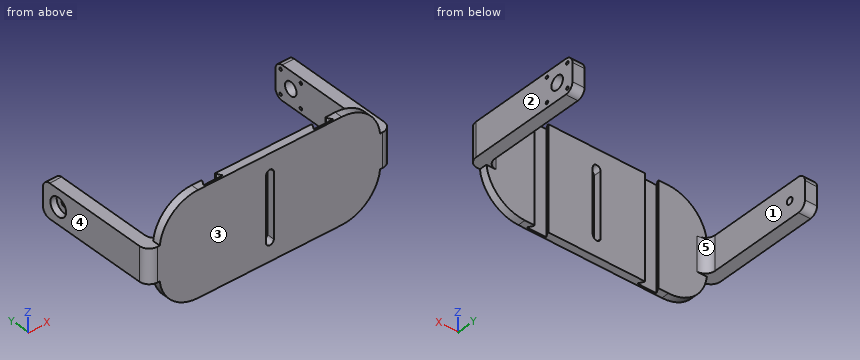
from build123d import *

# Parameters (mm, degrees)
SKETCH1_W           = 12.5
SKETCH1_H           = 127
BOSS_EXTRUDE1_DEPTH = 106
SKETCH2_W           = 12.5
SKETCH2_H           = 35.5
CUT_EXTRUDE1_DEPTH  = 200
SKETCH4_4_R         = 6
CUT_EXTRUDE3_DEPTH  = 37
SKETCH4_R           = 7
SKETCH4_R_2         = 1.55
CUT_EXTRUDE4_DEPTH  = 18.375
FILLET3_R           = 8
FILLET4_R           = 10
FILLET5_R           = 40
SKETCH5_R           = 3.5
CUT_EXTRUDE5_DEPTH  = 25
CUT_EXTRUDE6_START  = -6
SKETCH5_3_R         = 9.5
SKETCH5_3_R_2       = 3.5
CUT_EXTRUDE6_DEPTH  = 7


with BuildPart() as part:
    # Sketch1 → Boss-Extrude1 (new body)
    with BuildSketch(Plane.XY):
        Polygon((0, 8), (0, 0), (228, 0), (228, 8), (178.113248654, 8), (178.113248654, 7), (181, 2), (161, 2), (163.886751346, 7), (163.886751346, 8), (64.113248654, 8), (64.113248654, 7), (67, 2), (47, 2), (49.886751346, 7), (49.886751346, 8), align=None)
        with Locations((234.25, 63.5)):
            Rectangle(SKETCH1_W, SKETCH1_H)
        with Locations((-6.25, 63.5)):
            Rectangle(SKETCH1_W, SKETCH1_H)
    extrude(amount=-BOSS_EXTRUDE1_DEPTH)

    # Sketch2 → Cut-Extrude1 (cut)
    with BuildSketch(Plane(origin=(0, 127, 0), x_dir=(1, 0, 0), z_dir=(0, 1, 0))):
        with Locations((-6.25, 88.25)):
            Rectangle(SKETCH2_W, SKETCH2_H)
        with Locations((-6.25, 17.75)):
            Rectangle(SKETCH2_W, SKETCH2_H)
        with Locations((234.25, 88.25)):
            Rectangle(SKETCH2_W, SKETCH2_H)
        with Locations((234.25, 17.75)):
            Rectangle(SKETCH2_W, SKETCH2_H)
        with BuildLine():
            Line((109.95, 20), (109.95, 86))
            ThreePointArc((109.95, 86), (114, 90.05), (118.05, 86))
            Line((118.05, 86), (118.05, 20))
            ThreePointArc((118.05, 20), (114, 15.95), (109.95, 20))
        make_face()
    extrude(amount=-CUT_EXTRUDE1_DEPTH, mode=Mode.SUBTRACT)

    # Sketch4<4> → Cut-Extrude3 (cut)
    with BuildSketch(Plane(origin=(240.5, 0, 0), x_dir=(0, 0, -1), z_dir=(1, 0, 0))):
        with Locations((53, 108.5)):
            Circle(SKETCH4_4_R)
    extrude(amount=-CUT_EXTRUDE3_DEPTH, mode=Mode.SUBTRACT)

    # Sketch4 → Cut-Extrude4 (cut)
    with BuildSketch(Plane(origin=(240.5, 0, 0), x_dir=(0, 0, -1), z_dir=(1, 0, 0))):
        with Locations((53, 108.5)):
            Circle(SKETCH4_R)
        with Locations((40.625, 120.875)):
            Circle(SKETCH4_R_2)
        with Locations((40.625, 96.125)):
            Circle(SKETCH4_R_2)
        with Locations((65.375, 96.125)):
            Circle(SKETCH4_R_2)
        with Locations((65.375, 120.875)):
            Circle(SKETCH4_R_2)
    extrude(amount=-CUT_EXTRUDE4_DEPTH, mode=Mode.SUBTRACT)

    # Fillet3
    fillet3_edges = [part.edges().sort_by_distance(p)[0] for p in [
        (-6.25, 127, -35.5),
        (234.25, 127, -70.5),
        (234.25, 127, -35.5),
        (-6.25, 127, -70.5),
    ]]
    fillet(fillet3_edges, radius=FILLET3_R)

    # Fillet4
    fillet4_edges = [part.edges().sort_by_distance(p)[0] for p in [
        (228, 8, -53),
        (240.5, 0, -53),
        (0, 8, -53),
        (-12.5, 0, -53),
    ]]
    fillet(fillet4_edges, radius=FILLET4_R)

    # Fillet5
    # the kernel refuses this fillet: 40 mm, written as the material it takes off along each edge
    with BuildSketch(Plane(origin=(228, 107.36517247, -106), x_dir=(-1, 0, 0), z_dir=(0, -1, 0))) as fillet5_piece_1:
        with BuildLine():
            CenterArc((39.746068988, -40), FILLET5_R, 90, 83.540550223)
            Line((0, -35.5), (-0.79492138, -35.41))
            ThreePointArc((-0.79492138, -35.41), (-0.8, -17.75), (-0.8, 0))
            Line((-0.8, 0), (0, 0.8))
            Line((0, 0.8), (39.746068988, 0.8))
            Line((39.746068988, 0.8), (39.746068988, 0))
        make_face()
    extrude(amount=206.73034494, mode=Mode.SUBTRACT)
    with BuildSketch(Plane(origin=(0, 107.36517247, -106), x_dir=(0, 0, 1), z_dir=(0, -1, 0))) as fillet5_piece_2:
        with BuildLine():
            CenterArc((40, -39.746068988), FILLET5_R, 96.459449777, 83.540550223)
            Line((0, -39.746068988), (-0.8, -39.746068988))
            Line((-0.8, -39.746068988), (-0.8, 0))
            Line((-0.8, 0), (0, 0.8))
            ThreePointArc((0, 0.8), (17.75, 0.8), (35.41, 0.79492138))
            Line((35.41, 0.79492138), (35.5, 0))
        make_face()
    extrude(amount=206.73034494, mode=Mode.SUBTRACT)
    with BuildSketch(Plane(origin=(0, 107.36517247, 0), x_dir=(0, 0, -1), z_dir=(0, -1, 0))) as fillet5_piece_3:
        with BuildLine():
            CenterArc((40, 39.746068988), FILLET5_R, 180, 83.540550223)
            Line((0, 39.746068988), (-0.8, 39.746068988))
            Line((-0.8, 39.746068988), (-0.8, 0))
            Line((-0.8, 0), (0, -0.8))
            ThreePointArc((0, -0.8), (17.75, -0.8), (35.41, -0.79492138))
            Line((35.41, -0.79492138), (35.5, 0))
        make_face()
    extrude(amount=206.73034494, mode=Mode.SUBTRACT)
    with BuildSketch(Plane(origin=(228, 107.36517247, 0), x_dir=(-1, 0, 0), z_dir=(0, -1, 0))) as fillet5_piece_4:
        with BuildLine():
            CenterArc((39.746068988, 40), FILLET5_R, 186.459449777, 83.540550223)
            Line((0, 35.5), (-0.79492138, 35.41))
            ThreePointArc((-0.79492138, 35.41), (-0.8, 17.75), (-0.8, 0))
            Line((-0.8, 0), (0, -0.8))
            Line((0, -0.8), (39.746068988, -0.8))
            Line((39.746068988, -0.8), (39.746068988, 0))
        make_face()
    extrude(amount=206.73034494, mode=Mode.SUBTRACT)

    # Sketch5 → Cut-Extrude5 (cut)
    with BuildSketch(Plane(origin=(0, 0, 0), x_dir=(0, 0, -1), z_dir=(1, 0, 0))):
        with Locations((53, 108.5)):
            Circle(SKETCH5_R)
    extrude(amount=-CUT_EXTRUDE5_DEPTH, mode=Mode.SUBTRACT)

    # Sketch5<3> → Cut-Extrude6 (cut)
    with BuildSketch(Plane(origin=(0, 0, 0), x_dir=(0, 0, -1), z_dir=(1, 0, 0)).offset(CUT_EXTRUDE6_START)):
        with Locations((53, 108.5)):
            Circle(SKETCH5_3_R)
        with Locations((53, 108.5)):
            Circle(SKETCH5_3_R_2, mode=Mode.SUBTRACT)
    extrude(amount=-CUT_EXTRUDE6_DEPTH, mode=Mode.SUBTRACT)


solid = part.part
Geometry check sheet. Reference: the model listing, model coordinates, mm. Face numbers are marked on the shaded views. A direction names the side the tool comes from. Round coordinates to 2 decimals unless told otherwise and drop trailing zeros. Loops run counter-clockwise (first coordinate to the right, second up) from the corner with the lowest first, then second, coordinate; pieces in that order, holes last.
Item 1: Thickness scan on line 1 (Z direction, x = 233, y = 108); line 2 (X direction, y = 38, z = -65); line 3 (Y direction, x = 167, z = -45). Record the ranges inside material, lowest first.
Item 2: Cross-section at C-C on z = -74.5. Record the boundary of the cut face in (x, y), then the cut area to 3 significant figures.
Item 3: Access from +Z, -Z, +X, -X, +Y, -Y to the whole of each face (thin tool, end or side, straight path). Record for the marked faces 4 and 5.
Item 4: Cross-section at D-D on z = -53. Count the separate pieces of the cut face and the enclosed holes in it, then the cut area to 3 significant figures.
Item 5: Cross-section at A-A on y = 108.5. Record the boundary of the cut face in (x, z).
Item 6: Cross-section at B-B on x = 114. Record the boundary of the cut face in (y, z).
Item 7: Gauge pin test, flat ends, axial feed: pin 1 (15 mm diameter, centred on x = 207, z = -47, fed in from +Y); pin 2 (25 mm diameter, centred on x = 4, y = 75.5, fed in from -Z); pin 3 (6.5 mm diameter, centred on y = 108.5, z = -53, fed in from -X); pin 4 (18 mm diameter, centred on x = -1, y = 79, fed in from +Z). Record the tip position at first contact, or that the pin passes through.
Item 8: Mould release check, pull along X, two halves, no side actions. Record for the marked faces 1, 2 and 3: pulls with the +X half, pulls with the -X half, needs draft (parallel to the pull), parting line crosses it, or undercut.
Answer sheet:
1. line 1: z = -70.5 to -59.98, -46.02 to -35.5
1. line 2: x = -12.5 to 0, 228 to 240.5
1. line 3: y = 0 to 2
2. outline: (0.66, 0) - (109.95, 0) - (109.95, 8) - (64.11, 8) - (64.11, 7) - (67, 2) - (47, 2) - (49.89, 7) - (49.89, 8) - (0.66, 8) - close; (118.05, 0) - (227.34, 0) - (227.34, 8) - (178.11, 8) - (178.11, 7) - (181, 2) - (161, 2) - (163.89, 7) - (163.89, 8) - (118.05, 8) - close
2. area: 1,550 mm2
3. face 4: +Z, -Z, -X, +Y, -Y
3. face 5: +Z, -Z, +Y
4. separate pieces: 4
4. enclosed holes: 0
4. area: 4,390 mm2
5. outline: (-12.5, -70.5) - (0, -70.5) - (0, -56.5) - (-6, -56.5) - (-6, -62.5) - (-12.5, -62.5) - close; (-12.5, -43.5) - (-6, -43.5) - (-6, -49.5) - (0, -49.5) - (0, -35.5) - (-12.5, -35.5) - close; (228, -70.5) - (240.5, -70.5) - (240.5, -60) - (228, -60) - close; (228, -46) - (240.5, -46) - (240.5, -35.5) - (228, -35.5) - close
6. outline: (0, -106) - (8, -106) - (8, -90.05) - (0, -90.05) - close; (0, -15.95) - (8, -15.95) - (8, 0) - (0, 0) - close
7. pin 1: stops at y = 8
7. pin 2: stops at z = -70.5
7. pin 3: passes through
7. pin 4: stops at z = -35.5
8. face 1: undercut
8. face 2: pulls with the +X half
8. face 3: needs draft
